CAD build for the part. Positions are in the model's coordinates, mm. Face numbers are marked on the shaded views. A direction names the side the tool comes from. Coordinates: 2 decimals unless noted, no trailing zeros. Order: outer loops, then holes, each group sorted by start corner. A loop starts at its lowest first (then second) coordinate and runs counter-clockwise, first axis right, second up. Notation, with made-up numbers: M 89,61.5 L 129,61.5 A30 cw 129,95.5 Z; hole C -3.5,-24 d4. An arc over 180 degrees is marked long. One line per item, written item: value.
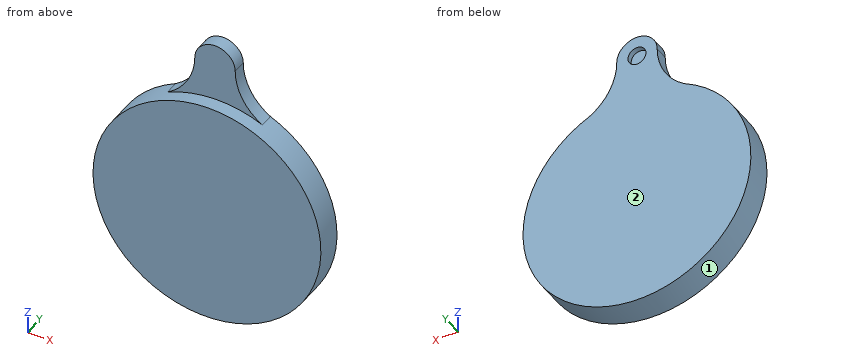
from build123d import *

# Parameters (mm, degrees)
SKETCH1_R           = 203
BOSS_EXTRUDE1_DEPTH = 50
BOSS_EXTRUDE2_START = -25
BOSS_EXTRUDE2_DEPTH = 25
SKETCH3_R           = 16
CUT_EXTRUDE1_DEPTH  = 10


with BuildPart() as part:
    # Sketch1 → Boss-Extrude1 (new body)
    with BuildSketch(Plane(origin=(0, 0, 0), x_dir=(1, 0, 0), z_dir=(0, 1, 0))):
        with Locations(Location((0, 0, 0), (0, 0, 270))):
            Circle(SKETCH1_R)
    extrude(amount=BOSS_EXTRUDE1_DEPTH)

    # Sketch2 → Boss-Extrude2 (add)
    with BuildSketch(Plane(origin=(0, 50, 0), x_dir=(1, 0, 0), z_dir=(0, 1, 0)).offset(BOSS_EXTRUDE2_START)):
        with BuildLine():
            ThreePointArc((-36, -270.29723777), (0, -306.29723777), (36, -270.29723777))
            ThreePointArc((36, -270.29723777), (48.967534793, -221.049395178), (84.507, -184.574014831))
            ThreePointArc((84.507, -184.574014831), (0, -203), (-84.507, -184.574014831))
            ThreePointArc((-84.507, -184.574014831), (-48.967534793, -221.049395178), (-36, -270.29723777))
        make_face()
    extrude(amount=BOSS_EXTRUDE2_DEPTH)

    # Sketch3 → Cut-Extrude1 (cut)
    with BuildSketch(Plane(origin=(0, 50, 0), x_dir=(1, 0, 0), z_dir=(0, 1, 0))):
        with Locations(Location((0, -270.29723777, 0), (0, 0, 270))):
            Circle(SKETCH3_R)
    extrude(amount=-CUT_EXTRUDE1_DEPTH, mode=Mode.SUBTRACT)


solid = part.part
Q1. Slice it at C-C (z = 209.5). List the corners of the cut face in (x, y), plus the area to 3 significant figures.
Recorded:
outline: M -56.6,25 L 56.6,25 L 56.6,50 L -56.6,50 Z
area: 2,830 mm^2
Q2. Slice it at A-A (x = 0). List the corners of the cut face in (y, z).
Recorded:
outline: M 0,-203 L 50,-203 L 50,254.3 L 40,254.3 L 40,286.3 L 50,286.3 L 50,306.3 L 25,306.3 L 25,203 L 0,203 Z
Q3. Slice it at B-B (y = 12). List the corners of the cut face in (x, z).
Recorded:
outline: C 0,0 d406
Q4. Which spindle directions (+Z, -Z, +X, -X, +Y, -Y) get a long thin tool onto all of the face, cutting with end or side? Do the marked faces 1 and 2. Say none if no direction does.
Recorded:
face 1: -Y
face 2: +Z, -Z, +X, -X, +Y
Q5. Slice it at D-D (x = 74). List the corners of the cut face in (y, z).
Recorded:
outline: M 0,-189.03 L 50,-189.03 L 50,191.84 L 25,191.84 L 25,189.03 L 0,189.03 Z
Q6. Pin check, flat tips, straight feed: pin 1 Ø10 at (x, y) = (99, 30.5) entering from +Z (3 decimals); pin 2 Ø4 at (x, y) = (11.5, 34) entering from -Z; pin 3 Ø6 at (x, y) = (73.5, 14.5) entering from +Z. Stop position of each tip, or through.
Recorded:
pin 1: stops at z = 179.925
pin 2: stops at z = -202.78
pin 3: stops at z = 190.36
Q7. Drill centre lines: line 1 along Z through (x, y) = (0.5, 10.5); line 2 along Y through (x, z) = (20, 279.5); line 3 along X through (y, z) = (19.5, 113.5). Where is each one in solid material? Low to high.
Recorded:
line 1: z = -203 to 203
line 2: y = 25 to 50
line 3: x = -168.31 to 168.31
